```python
from build123d import *

# Parameters (mm, degrees)
SKETCH1_W           = 206
SKETCH1_H           = 40
BOSS_EXTRUDE1_DEPTH = 20
SKETCH2_W           = 7.5
SKETCH2_H           = 40
BOSS_EXTRUDE2_DEPTH = 30
BOSS_EXTRUDE3_DEPTH = 206
CUT_EXTRUDE1_DEPTH  = 198.5
SKETCH7_R           = 7.9
CUT_EXTRUDE2_DEPTH  = 217.883289147


with BuildPart() as part:
    # Sketch1 → Boss-Extrude1 (new body)
    with BuildSketch(Plane.XY):
        with Locations((-0.375227687, 48.666666667)):
            Rectangle(SKETCH1_W, SKETCH1_H)
    extrude(amount=BOSS_EXTRUDE1_DEPTH)

    # Sketch2 → Boss-Extrude2 (add)
    with BuildSketch(Plane.XY.offset(20)):
        with Locations((98.874772313, 48.666666667)):
            Rectangle(SKETCH2_W, SKETCH2_H)
    extrude(amount=BOSS_EXTRUDE2_DEPTH)

    # Sketch4 → Boss-Extrude3 (add)
    with BuildSketch(Plane.ZY.offset(103.375227687)):
        with BuildLine():
            Line((7, 68.666666667), (13, 68.666666667))
            ThreePointArc((13, 68.666666667), (10, 71.666666667), (7, 68.666666667))
        make_face()
        with BuildLine():
            Line((7, 28.666666667), (13, 28.666666667))
            ThreePointArc((13, 28.666666667), (10, 25.666666667), (7, 28.666666667))
        make_face()
    extrude(amount=-BOSS_EXTRUDE3_DEPTH)

    # Sketch6 → Cut-Extrude1 (cut)
    with BuildSketch(Plane.ZY.offset(103.375227687)):
        Polygon((20, 56.666666667), (20, 60.666666667), (15, 60.666666667), (15, 63.666666667), (10, 63.666666667), (10, 53.666666667), (15, 53.666666667), (15, 56.666666667), align=None)
        Polygon((20, 36.666666667), (20, 40.666666667), (15, 40.666666667), (15, 43.666666667), (10, 43.666666667), (10, 33.666666667), (15, 33.666666667), (15, 36.666666667), align=None)
    extrude(amount=-CUT_EXTRUDE1_DEPTH, mode=Mode.SUBTRACT)

    # Sketch7 → Cut-Extrude2 (cut, through all)
    with BuildSketch(Plane.ZY.offset(-95.124772313)):
        with Locations(Location((35, 48.666666667, 0), (0, 0, 270))):
            Circle(SKETCH7_R)
    extrude(amount=-CUT_EXTRUDE2_DEPTH, mode=Mode.SUBTRACT)


solid = part.part
```
Here's how the part is built. I have some questions about the finished solid (model axes, mm). A direction names the side the tool comes from. Give positions to 0.01 mm unless a question says otherwise; leave off trailing zeros. Order: outer loops, then holes, each group sorted by start corner. A loop starts at its lowest first (then second) coordinate and runs counter-clockwise, first axis right, second up. Notation, with made-up numbers: M 29,2.5 L 60,2.5 A16 cw 60,26.5 Z; hole C 87.25,2.25 d6. An arc over 180 degrees is marked long. Use a Markdown table: item, result. Add a question column.
1. For pin 1 Ø2 at (x, z) = (14.5, 4) entering from -Y; pin 2 Ø2 at (y, z) = (59.5, 23) entering from -X; pin 3 Ø1.5 at (x, y) = (42, 55) entering from -Z; pin 4 Ø11 at (x, y) = (-26.5, 58) entering from +Z, each with a flat end and sliding along its axis, tell me the tip position at first contact or that it passes through.
2. Suppose I cut it at D-D (y = 66). List the corners of the cut face in (x, z) for me.
3. I need wall thicknesses on probe 1 along Y at (x, z) = (12.5, 15.5); probe 2 along Z at (x, y) = (44, 56); probe 3 along Y at (x, z) = (67, 12). Which ranges of each line are inside material? Lowest first, please. Write a range as from..to.
4. Suppose I cut it at A-A (z = 35). List the corners of the cut face in (x, y) for me, and give its area (4 significant figures).
5. Suppose I cut it at B-B (x = 75.5). List the corners of the cut face in (y, z) for me, and give its area (3 significant figures).
6. On a 3-axis mill with a long thin cutter (end or side, diameter ignored), from which of +Z, -Z, +X, -X, +Y, -Y can I reach the whole of each face in a straight line? I mean faces 4 (the flat face through (-6, 36.667, 17)), 5 (the flat face through (-6, 53.667, 12)), 6 (the flat face through (-2, 28.667, 3)). Say none if no direction works.
7. Suppose I cut it at C-C (z = 17). List the corners of the cut face in (x, y) for me, and give its area (3 significant figures).
8. If we mould it in two halves opening along Y, with no side actions, what happens to faces 1 (the flat face through (-6, 43.667, 13)), 2 (the flat face through (-6, 65, 20)), 3 (the flat face through (14, 28.667, 19))? For each: +Y half, -Y half, draft (parallel to the pull), parting line (faces both ways), or undercut.
Results list:
| question | item | result |
|---|---|---|
| 1 | pin 1 | stops at y = 28.67 |
| 1 | pin 2 | stops at x = 95.12 |
| 1 | pin 3 | stops at z = 0 |
| 1 | pin 4 | stops at z = 20 |
| 2 | outline | M -103.38,0 L 102.62,0 L 102.62,50 L 95.12,50 L 95.12,20 L -103.38,20 Z |
| 3 | probe 1 | y = 28.67..36.67, 40.67..56.67, 60.67..68.67 |
| 3 | probe 2 | z = 0..10, 15..20 |
| 3 | probe 3 | y = 26.43..33.67, 43.67..53.67, 63.67..70.9 |
| 4 | outline | M 95.12,28.67 L 102.62,28.67 L 102.62,40.77 L 95.12,40.77 Z; M 95.12,56.57 L 102.62,56.57 L 102.62,68.67 L 95.12,68.67 Z |
| 4 | area | 181.5 mm² |
| 5 | outline | M 28.67,0 L 68.67,0 L 68.67,7 A3 ccw 68.67,13 L 68.67,20 L 60.67,20 L 60.67,15 L 63.67,15 L 63.67,10 L 53.67,10 L 53.67,15 L 56.67,15 L 56.67,20 L 40.67,20 L 40.67,15 L 43.67,15 L 43.67,10 L 33.67,10 L 33.67,15 L 36.67,15 L 36.67,20 L 28.67,20 L 28.67,13 A3 ccw 28.67,7 Z |
| 5 | area | 688 mm² |
| 6 | face 4 | +Z, -X |
| 6 | face 5 | -X |
| 6 | face 6 | -Z, +X, -X, -Y |
| 7 | outline | M -103.38,28.67 L 102.62,28.67 L 102.62,68.67 L -103.38,68.67 L -103.38,60.67 L 95.12,60.67 L 95.12,56.67 L -103.38,56.67 L -103.38,40.67 L 95.12,40.67 L 95.12,36.67 L -103.38,36.67 Z |
| 7 | area | 6,650 mm² |
| 8 | face 1 | undercut |
| 8 | face 2 | draft |
| 8 | face 3 | -Y half |
